```python
from build123d import *

# Parameters (mm, degrees)
F0_W      = 63.8
F0_H      = 31.8
F0_W_2    = 60.8
F0_H_2    = 28.8
F1_DEPTH  = 12.8
F2_W      = 6.3
F2_H      = 6.3
F2_W_2    = 7.8
F3_DEPTH  = 1
F4_R      = 2.45
F5_DEPTH  = 1.8
F6_W      = 0.85
F6_H      = 0.5
F7_DEPTH  = 25.4
F9_DEPTH  = 8
F11_DEPTH = 5
F12_W     = 0.1
F12_H     = 1
F13_DEPTH = 6.3
F14_W     = 6
F14_H     = 1.7
F15_DEPTH = 2.54
F16_W     = 11
F16_H     = 6
F16_W_2   = 6
F16_H_2   = 1.7
F17_DEPTH = 0.5
F19_DEPTH = 5
F21_DEPTH = 4
F23_DEPTH = 25.4


# Not quite as in the source:
# - a feature names something its author has since deleted; it is built from what else it names


with BuildPart() as f1:
    # F0 (on Top) → F1 (new body)
    with BuildSketch(Plane.XY):
        with Locations((31.9, 15.9)):
            Rectangle(F0_W, F0_H)
        with Locations((31.9, 15.9)):
            Rectangle(F0_W_2, F0_H_2, mode=Mode.SUBTRACT)
    extrude(amount=F1_DEPTH)

    # F2 (on face) → F3 (join)
    with BuildSketch(Plane.XY.offset(12.8)):
        with Locations((4.65, 27.15)):
            Rectangle(F2_W, F2_H)
        with Locations((4.65, 4.65)):
            Rectangle(F2_W, F2_H)
        with Locations((59.15, 4.65)):
            Rectangle(F2_W, F2_H)
        with Locations((59.15, 27.15)):
            Rectangle(F2_W, F2_H)
        with Locations((27.9, 27.15)):
            Rectangle(F2_W_2, F2_H)
        with Locations((35.9, 4.65)):
            Rectangle(F2_W_2, F2_H)
    extrude(amount=-F3_DEPTH)

    # F4 (on face) → F5 (join)
    with BuildSketch(Plane.XY.offset(12.8)):
        with Locations((3.9, 27.9)):
            Circle(F4_R)
        with Locations((59.9, 27.9)):
            Circle(F4_R)
        with Locations((59.9, 3.9)):
            Circle(F4_R)
        with Locations((3.9, 3.9)):
            Circle(F4_R)
        with Locations((27.9, 27.9)):
            Circle(F4_R)
        with Locations((35.9, 3.9)):
            Circle(F4_R)
    extrude(amount=F5_DEPTH)

    # F6 (on face) → F7 (cut)
    with BuildSketch(Plane.XZ):
        Polygon((11.575, 10.95), (9.7, 10.95), (9.7, 7.15), (14.3, 7.15), (14.3, 10.95), (12.425, 10.95), align=None)
        with Locations((12, 11.2)):
            Rectangle(F6_W, F6_H)
    extrude(amount=-F7_DEPTH, mode=Mode.SUBTRACT)

    # F8 (on face) → F9 (join)
    with BuildSketch(Plane(origin=(0, 1.5, 0), x_dir=(-1, 0, 0), z_dir=(0, 1, 0))):
        Polygon((-13.6, 5.8), (-13.6, 6.8), (-15.1, 6.8), (-15.1, 11.8), (-13.6, 11.8), (-13.6, 12.8), (-16.1, 12.8), (-16.1, 5.8), align=None)
        Polygon((-8.9, 6.8), (-10.4, 6.8), (-10.4, 5.8), (-7.9, 5.8), (-7.9, 12.8), (-10.4, 12.8), (-10.4, 11.8), (-8.9, 11.8), align=None)
    extrude(amount=F9_DEPTH)

    # F10 (on face) → F11 (join, through all)
    with BuildSketch(Plane.XY.offset(6.8)):
        Polygon((14.6, 7.6), (15.1, 7.6), (15.1, 9.5), align=None)
        Polygon((9.4, 7.6), (8.9, 9.5), (8.9, 7.6), align=None)
    extrude(amount=F11_DEPTH)

    # F12 (on face) → F13 (join, through all)
    with BuildSketch(Plane(origin=(0, 1.5, 0), x_dir=(-1, 0, 0), z_dir=(0, 1, 0))):
        with Locations((-7.85, 12.3)):
            Rectangle(F12_W, F12_H)
    extrude(amount=F13_DEPTH)

    # F14 (on face) → F15 (cut)
    with BuildSketch(Plane(origin=(0, 31.8, 0), x_dir=(-1, 0, 0), z_dir=(0, 1, 0))):
        with Locations((-12, 6.4)):
            Rectangle(F14_W, F14_H)
    extrude(amount=-F15_DEPTH, mode=Mode.SUBTRACT)

    # F16 (on face) → F17 (join)
    with BuildSketch(Plane.XZ.offset(-30.3)):
        with Locations((12, 6.4)):
            Rectangle(F16_W, F16_H)
        with Locations((12, 6.4)):
            Rectangle(F16_W_2, F16_H_2, mode=Mode.SUBTRACT)
    extrude(amount=F17_DEPTH)

    # F18 (on face) → F19 (join)
    with BuildSketch(Plane.XZ.offset(-29.8)):
        Polygon((9, 9.4), (6.5, 9.4), (6.5, 3.4), (9, 3.4), (9, 4.4), (7.5, 4.4), (7.5, 8.4), (9, 8.4), align=None)
        Polygon((17.5, 9.4), (15, 9.4), (15, 8.4), (16.5, 8.4), (16.5, 4.4), (15, 4.4), (15, 3.4), (17.5, 3.4), align=None)
    extrude(amount=F19_DEPTH)

    # F20 (on face) → F21 (join, through all)
    with BuildSketch(Plane.XY.offset(4.4)):
        Polygon((7.5, 25.8), (7.5, 24.8), (8, 25.8), align=None)
        Polygon((16, 25.8), (16.5, 24.8), (16.5, 25.8), align=None)
    extrude(amount=F21_DEPTH)

    # F22 (on face) → F23 (cut)
    with BuildSketch(Plane(origin=(0, 0, 0), x_dir=(0, -1, 0), z_dir=(-1, 0, 0))):
        with BuildLine():
            Line((-13.8921684574, 8.65), (-17.9078315426, 8.65))
            ThreePointArc((-17.9078315426, 8.65), (-18.3088802049, 8.4838802049), (-18.475, 8.0828315426))
            Line((-18.475, 8.0828315426), (-18.475, 4.7171684574))
            ThreePointArc((-18.475, 4.7171684574), (-18.3088802049, 4.3161197951), (-17.9078315426, 4.15))
            Line((-17.9078315426, 4.15), (-13.8921684574, 4.15))
            ThreePointArc((-13.8921684574, 4.15), (-13.4911197951, 4.3161197951), (-13.325, 4.7171684574))
            Line((-13.325, 4.7171684574), (-13.325, 8.0828315426))
            ThreePointArc((-13.325, 8.0828315426), (-13.4911197951, 8.4838802049), (-13.8921684574, 8.65))
        make_face()
    extrude(amount=-F23_DEPTH, mode=Mode.SUBTRACT)


solid = f1.part
```
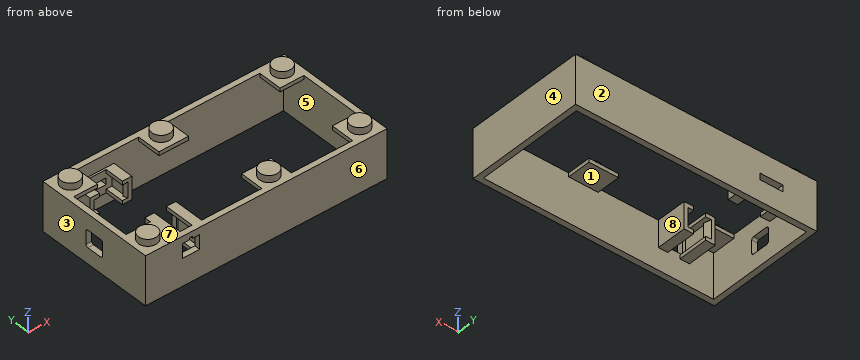
Input: part model. Units: mm. Frame: model coordinates. Face numbers are marked on the shaded views. A direction names the side the tool comes from. Give positions to 0.01 mm unless a question says otherwise; leave off trailing zeros. Order: outer loops, then holes, each group sorted by start corner. A loop starts at its lowest first (then second) coordinate and runs counter-clockwise, first axis right, second up. Notation, with made-up numbers: M 20,-19.5 L 75,-19.5 A30 ccw 75,2.5 Z; hole C 25,45 d5. An arc over 180 degrees is marked long. Return JSON: item names as keys, results as strings.
Item 1: Cut plane B-B (x = 20.5). Return loops of the section in (y, z).
Solutions:
{"outline": "M 0,0 L 1.5,0 L 1.5,12.8 L 0,12.8 Z; M 30.3,0 L 31.8,0 L 31.8,12.8 L 30.3,12.8 Z"}
Item 2: Pull-direction query (Y, two-part tool) for the marked faces 1, 2 and 3; classes: +Y half, -Y half, draft (parallel to the pull), parting line (faces both ways), or undercut.
Solutions:
{"face 1": "undercut", "face 2": "+Y half", "face 3": "draft"}
Item 3: Cut plane D-D (x = 3.9). Return loops of the section in (y, z), then the cut area to 3 significant figures.
Solutions:
{"outline": "M 0,0 L 1.5,0 L 1.5,11.8 L 7.8,11.8 L 7.8,12.8 L 6.35,12.8 L 6.35,14.6 L 1.45,14.6 L 1.45,12.8 L 0,12.8 Z; M 24,11.8 L 30.3,11.8 L 30.3,0 L 31.8,0 L 31.8,12.8 L 30.35,12.8 L 30.35,14.6 L 25.45,14.6 L 25.45,12.8 L 24,12.8 Z", "area": "68.6 mm^2"}
Item 4: Cut plane A-A (z = 1.75). Return loops of the section in (x, y), then the cut area to 3 significant figures.
Solutions:
{"outline": "M 0,0 L 63.8,0 L 63.8,31.8 L 0,31.8 Z; hole M 1.5,1.5 L 62.3,1.5 L 62.3,30.3 L 1.5,30.3 Z", "area": "278 mm^2"}
Item 5: Access query for the marked faces 4, 5, 6, 7 and 8. Directions: +Z, -Z, +X, -X, +Y, -Y. A direction counts if a zero-diameter tool reaches every point of the face in a straight line with its end or side. Return the directions, or none.
Solutions:
{"face 4": "+Z, -Z, +X, +Y, -Y", "face 5": "-Z", "face 6": "+Z, -Z, +X, -X, -Y", "face 7": "+Z", "face 8": "+Z, -Z"}
Item 6: First-contact query: P1, Ø0.8, axis at x = 9.5, y = 5, coming from the +Z side; P2, Ø1.2, axis at x = 0.5, z = 6, coming from the -Y side; P3, Ø1.6, axis at x = 9.5, y = 4.5, coming from the -Z side; P4, Ø4.5, axis at x = 10, y = 27, coming from the -Z side. Flat tips, straight axial feed; report the tip coordinate or a pass-through.
Solutions:
{"P1": "z = 12.8", "P2": "y = 0", "P3": "z = 5.8", "P4": "z = 3.4"}
Item 7: Cut plane C-C (y = 21). Return loops of the section in (x, z), then the cut area to 3 significant figures.
Solutions:
{"outline": "M 0,0 L 1.5,0 L 1.5,12.8 L 0,12.8 Z; M 62.3,0 L 63.8,0 L 63.8,12.8 L 62.3,12.8 Z", "area": "38.4 mm^2"}
Item 8: Ray query, probe 1 along X at (y, z) = (27.5, 7.25); probe 2 along X at (y, z) = (5, 6); probe 3 along Y at (x, z) = (34, 6.25). Return the intervals inside material, ascending.
Solutions:
{"probe 1": "0 to 1.5, 6.5 to 7.5, 16.5 to 17.5, 62.3 to 63.8", "probe 2": "0 to 1.5, 7.9 to 10.4, 13.6 to 16.1, 62.3 to 63.8", "probe 3": "0 to 1.5, 30.3 to 31.8"}
